Input: part model. Units: mm. Frame: model coordinates. Face numbers are marked on the shaded views. Coordinates: 2 decimals unless noted, no trailing zeros. Order: outer loops, then holes, each group sorted by start corner. A loop starts at its lowest first (then second) coordinate and runs counter-clockwise, first axis right, second up. Notation, with made-up numbers: (-12, -9.5) -> (2, -9.5) arc R17 ccw to (2, 7.5) -> close; hole circle Ø6 at (-6, -3.5). An arc over 180 degrees is marked (long way). Answer as CSV lines item,"result".
from build123d import *

# Parameters (mm, degrees)
BOSS_EXTRUDE1_DEPTH = 6.35
SKETCH2_W           = 6.35
SKETCH2_H           = 12.7
BOSS_EXTRUDE2_DEPTH = 6.35
LPATTERN1_COUNT     = 2
LPATTERN1_PITCH     = 63.5
SKETCH3_R           = 1.25
SKETCH3_R_2         = 6
CUT_EXTRUDE1_DEPTH  = 93.937051949
SKETCH4_W           = 6.35
SKETCH4_H           = 12.7
SKETCH4_H_2         = 12.666633789
BOSS_EXTRUDE3_DEPTH = 6.35
CUT_EXTRUDE2_DEPTH  = 98.221400036


with BuildPart() as part:
    # Sketch1 → Boss-Extrude1 (new body)
    with BuildSketch(Plane.XY):
        Polygon((-60.975, 31.75), (21.575, 31.75), (21.575, -38.788945114), (21.575, -69.85), (15.225, -69.85), (-60.975, -38.788945114), align=None)
    extrude(amount=BOSS_EXTRUDE1_DEPTH)

    # Sketch2 → Boss-Extrude2 (add)
    with BuildSketch(Plane(origin=(21.575, 0, 0), x_dir=(0, 0, -1), z_dir=(1, 0, 0))):
        with Locations((-3.175, -63.5)):
            Rectangle(SKETCH2_W, SKETCH2_H)
    boss_extrude2 = extrude(amount=BOSS_EXTRUDE2_DEPTH)

    # LPattern1: Boss-Extrude2 ×2
    with Locations(*[(0, i * LPATTERN1_PITCH, 0) for i in range(1, LPATTERN1_COUNT)]):
        add(boss_extrude2)

    # Sketch3 → Cut-Extrude1 (cut, through all)
    with BuildSketch(Plane(origin=(0, 0, 0), x_dir=(-1, 0, 0), z_dir=(0, 0, -1))):
        with Locations((13.423393759, 7.75)):
            Circle(SKETCH3_R)
        with Locations((13.423393759, -7.75)):
            Circle(SKETCH3_R)
        with Locations((0, 15.5)):
            Circle(SKETCH3_R)
        with Locations((-13.423393759, 7.75)):
            Circle(SKETCH3_R)
        with Locations((-13.423393759, -7.75)):
            Circle(SKETCH3_R)
        with Locations((0, -15.5)):
            Circle(SKETCH3_R)
        with Locations((-7, 0)):
            Circle(SKETCH3_R_2)
    extrude(amount=-CUT_EXTRUDE1_DEPTH, mode=Mode.SUBTRACT)

    # Sketch4 → Boss-Extrude3 (add)
    with BuildSketch(Plane.ZY.offset(60.975)):
        with Locations((3.175, 25.4)):
            Rectangle(SKETCH4_W, SKETCH4_H)
        with Locations((3.175, -25.416683106)):
            Rectangle(SKETCH4_W, SKETCH4_H_2)
    extrude(amount=BOSS_EXTRUDE3_DEPTH)

    # Sketch5 → Cut-Extrude2 (cut, through all)
    with BuildSketch(Plane.XY.offset(6.35)):
        Polygon((-60.975, 2.0955), (-60.975, -2.0955), (-52.212, -2.0955), (-52.212, -3.429), (-49.672, -3.429), (-49.672, -2.0955), (-46.37, -2.0955), (-46.37, 2.0955), (-49.672, 2.0955), (-49.672, 3.429), (-52.212, 3.429), (-52.212, 2.0955), align=None)
        Polygon((21.575, -52.8955), (21.575, -48.7045), (12.812, -48.7045), (12.812, -47.371), (10.272, -47.371), (10.272, -48.7045), (6.97, -48.7045), (6.97, -52.8955), (10.272, -52.8955), (10.272, -54.229), (12.812, -54.229), (12.812, -52.8955), align=None)
        Polygon((21.575, 16.9545), (21.575, 21.1455), (12.812, 21.1455), (12.812, 22.479), (10.272, 22.479), (10.272, 21.1455), (6.97, 21.1455), (6.97, 16.9545), (10.272, 16.9545), (10.272, 15.621), (12.812, 15.621), (12.812, 16.9545), align=None)
    extrude(amount=-CUT_EXTRUDE2_DEPTH, mode=Mode.SUBTRACT)


solid = part.part
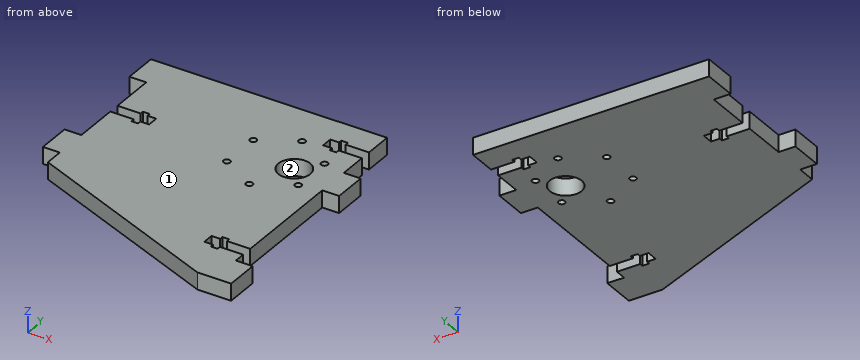
1. Cut plane B-B (z = 2.25). State how many separate pieces and enclosed holes the cut face has, plus the area to 3 significant figures.
Findings:
separate pieces,"1"
enclosed holes,"7"
area,"7,180 mm2"
2. Contact query for flat-ended pins moving along their axis: pin 1 (2 mm diameter, centred on y = -14.5, z = 5.5, fed in from -X) (3 decimals); pin 2 (1.5 mm diameter, centred on x = 0, y = 15.5, fed in from +Z); pin 3 (2 mm diameter, centred on x = 11.5, z = 3.5, fed in from -Y); pin 4 (6 mm diameter, centred on x = -35.5, y = -47.5, fed in from -Z). Output: stop coordinate, or through.
Findings:
pin 1,"stops at x = -60.975"
pin 2,"passes through"
pin 3,"stops at y = -68.74"
pin 4,"stops at z = 0"
3. Cut plane D-D (y = -40). Return the cut outline in (x, z) (3 decimals).
Findings:
outline,"(-58.004, 0) -> (21.575, 0) -> (21.575, 6.35) -> (-58.004, 6.35) -> close"
4. Mould query, pull axis X, two halves, no side actions, for the marked faces 1 and 2. Classes: released by +X, released by -X, zero draft, split by the parting line, or undercut.
Findings:
face 1,"zero draft"
face 2,"undercut"
5. Cut plane A-A (y = -7.75). Return the cut outline in (x, z) (3 decimals), plus the area to 3 significant figures.
Findings:
outline,"(-60.975, 0) -> (-14.673, 0) -> (-14.673, 6.35) -> (-60.975, 6.35) -> close; (-12.173, 0) -> (12.173, 0) -> (12.173, 6.35) -> (-12.173, 6.35) -> close; (14.673, 0) -> (21.575, 0) -> (21.575, 6.35) -> (14.673, 6.35) -> close"
area,"492 mm2"
6. Cut plane C-C (x = -28.5). Return the cut outline in (y, z).
Findings:
outline,"(-52.03, 0) -> (31.75, 0) -> (31.75, 6.35) -> (-52.03, 6.35) -> close"
7. Ray query, line 1 along Y through (x, z) = (-1, 0.75); line 2 along Y through (x, z) = (0, 2.25); line 3 along X through (y, z) = (17.5, 0.5) (3 decimals). Return the intervals inside material, ascending.
Findings:
line 1,"y = -63.24 to -16.25, -14.75 to 14.75, 16.25 to 31.75"
line 2,"y = -63.64 to -16.75, -14.25 to 14.25, 16.75 to 31.75"
line 3,"x = -60.975 to 6.97"
